Design review of the part built by this model. Coordinates are the model's own, in mm. A direction names the side the tool comes from. Give positions to 0.01 mm unless a question says otherwise; leave off trailing zeros. Write each loop counter-clockwise with the first axis right and the second up, starting at its lowest first coordinate (ties: lowest second). Pieces come first, ordered by that corner, then holes. Notation, with made-up numbers: (86, -37.5) -> (131, -37.5) arc R18 ccw to (131, -8.5) -> close; hole circle Ø6 at (31, -26). An arc over 180 degrees is marked (long way). Put each result on its own line as item: value. Start each with the question number.
from build123d import *

# Parameters (mm, degrees)
BOSS_EXTRUDE1_DEPTH      = 4
BOSS_EXTRUDE1_DEPTH_BACK = 2
SKETCH2_W                = 10
SKETCH2_H                = 5
BOSS_EXTRUDE2_DEPTH      = 50
FILLET1_RADIUS           = 5
FILLET1_LENGTH           = 5
SKETCH3_R                = 2.7
CUT_EXTRUDE1_DEPTH       = 35
BOSS_EXTRUDE3_DEPTH      = 5
BOSS_EXTRUDE5_START      = -5
BOSS_EXTRUDE5_DEPTH      = 10


# Read off the part's stored shape, not the designer's step: Boss-Extrude5
with BuildPart() as part:
    # Sketch1 → Boss-Extrude1 (new, two sides: drawn at the far end of the back side and taken through both)
    with BuildSketch(Plane.XY.offset(-BOSS_EXTRUDE1_DEPTH_BACK)):
        with BuildLine():
            Line((-35, -25), (35, -25))
            Line((35, -25), (35, 25))
            Line((35, 25), (22, 25))
            ThreePointArc((22, 25), (0, 3), (-22, 25))
            Line((-22, 25), (-35, 25))
            Line((-35, 25), (-35, -25))
        make_face()
    extrude(amount=BOSS_EXTRUDE1_DEPTH + BOSS_EXTRUDE1_DEPTH_BACK)

    # Sketch2 → Boss-Extrude2 (add)
    with BuildSketch(Plane.XY.offset(4)):
        with Locations((0, -11)):
            Rectangle(SKETCH2_W, SKETCH2_H)
    extrude(amount=BOSS_EXTRUDE2_DEPTH)

    # Fillet1: full round fillet: the end face becomes a half cylinder, R = half its width
    fillet1_face = Plane((0, -11, 54), x_dir=(0, -1, 0), z_dir=(0, 0, 1))  # on the end face: x along it, z out of the body
    fillet1_slab = fillet1_face.offset(-FILLET1_RADIUS / 2) * Box(FILLET1_LENGTH, 2 * FILLET1_RADIUS, FILLET1_RADIUS, mode=Mode.PRIVATE)  # the body's end, R deep
    fillet1_round = Plane((0, -11, 49), x_dir=(0, 0, 1), z_dir=(0, -1, 0)) * Cylinder(FILLET1_RADIUS, FILLET1_LENGTH, mode=Mode.PRIVATE)  # its axis R under the face
    add(fillet1_slab - fillet1_round, mode=Mode.SUBTRACT)

    # Sketch3 → Cut-Extrude1 (cut)
    with BuildSketch(Plane(origin=(0, -8.5, 0), x_dir=(1, 0, 0), z_dir=(0, 1, 0))):
        with Locations(Location((0, -49, 0), (0, 0, 180))):
            Circle(SKETCH3_R)
    extrude(amount=-CUT_EXTRUDE1_DEPTH, mode=Mode.SUBTRACT)

    # Sketch6 → Boss-Extrude3 (add)
    with BuildSketch(Plane.XZ.offset(13.5)):
        with BuildLine():
            Line((5, 4), (20, 4))
            ThreePointArc((20, 4), (9.393398282, 8.393398282), (5, 19))
            Line((5, 19), (5, 4))
        make_face()
        with BuildLine():
            Line((-5, 4), (-20, 4))
            ThreePointArc((-20, 4), (-9.393398282, 8.393398282), (-5, 19))
            Line((-5, 19), (-5, 4))
        make_face()
    extrude(amount=-BOSS_EXTRUDE3_DEPTH)

    # Boss-Extrude5 outline → Boss-Extrude5 (add)
    with BuildSketch(Plane(origin=(0, 0, 0), x_dir=(0, 0, -1), z_dir=(1, 0, 0)).offset(BOSS_EXTRUDE5_START)):
        with BuildLine():
            ThreePointArc((-13.190244239, -13.5), (-6.643691612, -17.19601893), (-4, -24.233689133))
            Line((-4, -24.233689133), (-4, -13.5))
            Line((-4, -13.5), (-13.190244239, -13.5))
        make_face()
    extrude(amount=BOSS_EXTRUDE5_DEPTH)


solid = part.part
Q1. Take a section at B-B on y = -12. Give the boundary of the cut face in (x, z), then the cut area to 3 significant figures.
Q2. Take a section at C-C on z = 22.5. Give the boundary of the cut face in (x, y).
Q3. For pin 1 (6 mm diameter, centred on y = -9, z = 36, fed in from -X); pin 2 (12 mm diameter, centred on x = 6, z = 29.5, fed in from +Y); pin 3 (12 mm diameter, centred on y = -15.5, z = 35, fed in from +X), all flat-tipped, find the tip position at first contact; note any pin that passes through.
Q4. Mouldability with a two-part tool opening along X and no side actions: class faces 4 (the face through (-35, 0, 1)), 5 (the face through (-1.246, -10.965, 46.605)), 6 (the face through (0, -13.5, 29)) as +X half, -X half, draft (parallel to the pull), parting line (faces both ways), or undercut.
Q5. Machinability: for faces 1 (the face through (0, -8.5, 24)), 2 (the face through (0, -5, 4)), 3 (the face through (-5, -16, 6)), which of the approach directions +Z, -Z, +X, -X, +Y, -Y give a long, thin tool a straight path to every point of the face, cutting with its end or side? Answer none if there is none.
Q6. To check wall thickness, follow probe 1 along Z at (x, y) = (0, -10.2); probe 2 along Z at (x, y) = (-20, -13); probe 3 along Y at (x, z) = (-2, 33). State the ranges of each line that lie inside material, in increasing order. Write a range as from..to.
Q7. Take a section at D-D on z = 10. Give the boundary of the cut face in (x, y).
Q8. Take a section at A-A on x = 0. Give the boundary of the cut face in (y, z), then the cut area to 3 significant figures.
Result:
1. outline: (-35, -2) -> (35, -2) -> (35, 4) -> (20, 4) arc R15 cw to (5, 19) -> (5, 49) arc R5 ccw to (-5, 49) -> (-5, 19) arc R15 cw to (-20, 4) -> (-35, 4) -> close; hole circle Ø5.4 at (0, 49)
1. area: 983 mm^2
2. outline: (-5, -13.5) -> (5, -13.5) -> (5, -8.5) -> (-5, -8.5) -> close
3. pin 1: stops at x = -5
3. pin 2: stops at y = -8.5
3. pin 3: stops at x = 5
4. face 4: -X half
4. face 5: undercut
4. face 6: draft
5. face 1: +Z, +X, -X, +Y
5. face 2: +Z
5. face 3: +Z, -X, -Y
6. probe 1: z = -2..46.3, 51.7..54
6. probe 2: z = -2..4
6. probe 3: y = -13.5..-8.5
7. outline: (-8, -13.5) -> (-5, -13.5) -> (-5, -14.55) -> (5, -14.55) -> (5, -13.5) -> (8, -13.5) -> (8, -8.5) -> (-8, -8.5) -> close
8. outline: (-25, -2) -> (3, -2) -> (3, 4) -> (-8.5, 4) -> (-8.5, 46.3) -> (-13.5, 46.3) -> (-13.5, 13.19) arc R11 cw to (-24.23, 4) -> (-25, 4) -> close; (-13.5, 51.7) -> (-8.5, 51.7) -> (-8.5, 54) -> (-13.5, 54) -> close
8. area: 415 mm^2
